The listing builds one solid part. Answer for the finished solid, in the listing's coordinates (mm). A direction names the side the tool comes from. Coordinates: 2 decimals unless noted, no trailing zeros. Loops run counter-clockwise (first coordinate to the right, second up) from the corner with the lowest first, then second, coordinate; pieces in that order, holes last. Notation, with made-up numbers: (-20.75, 32.25) -> (11.25, 32.25) arc R32 cw to (11.25, 68.25) -> close; hole circle Ø2 at (52.25, 55). An arc over 180 degrees is marked (long way). Answer in a Markdown table with one row per item.
```python
from build123d import *

# Parameters (mm, degrees)
F0_W      = 203.2
F0_H      = 203.2
F1_DEPTH  = 203.2
F2_W      = 198.12
F2_H      = 198.12
F3_DEPTH  = 200.66
F7_DEPTH  = 203.201
F10_DEPTH = 2.54
F13_DEPTH = 2.54


with BuildPart() as f1:
    # F0 (on Top) → F1 (new body)
    with BuildSketch(Plane.XY):
        Rectangle(F0_W, F0_H)
    extrude(amount=F1_DEPTH)

    # F2 (on Top) → F3 (cut)
    with BuildSketch(Plane.XY):
        Rectangle(F2_W, F2_H)
    extrude(amount=F3_DEPTH, mode=Mode.SUBTRACT)

    # F6 (on offset) → F7 (cut, through all)
    with BuildSketch(Plane.YZ.offset(101.6)):
        Polygon((1.27, 76.2), (1.27, 101.6), (-99.06, 101.6), (-99.06, 0), (99.06, 0), (99.06, 76.2), align=None)
    extrude(amount=-F7_DEPTH, mode=Mode.SUBTRACT)

    # F9 (on offset) → F10 (cut, through all)
    with BuildSketch(Plane(origin=(0, 101.6, 0), x_dir=(-1, 0, 0), z_dir=(0, 1, 0))):
        Polygon((-101.6, 0), (101.6, 0), (101.6, 25.4), (101.6, 50.8), (50.8, 50.8), (50.8, 25.4), (-50.8, 25.4), (-50.8, 50.8), (-101.6, 50.8), (-101.6, 25.4), align=None)
    extrude(amount=-F10_DEPTH, mode=Mode.SUBTRACT)

    # F12 (on offset) → F13 (cut, through all)
    with BuildSketch(Plane.XZ.offset(101.6)):
        Polygon((-101.6, 101.6), (-101.6, 0), (101.6, 0), (101.6, 101.6), (76.2, 101.6), (76.2, 127), (25.4, 127), (25.4, 101.6), (25.4, 76.2), (-25.4, 76.2), (-25.4, 101.6), (-25.4, 127), (-76.2, 127), (-76.2, 101.6), align=None)
    extrude(amount=-F13_DEPTH, mode=Mode.SUBTRACT)


solid = f1.part
```
Item 1: A cutting plane is placed at B-B, the plane x = 87.5. Determine the outline of the cut face in (y, z), plus the area to 3 significant figures.
Findings below:
| item | result |
|---|---|
| outline | (-101.6, 101.6) -> (-99.06, 101.6) -> (-99.06, 200.66) -> (99.06, 200.66) -> (99.06, 50.8) -> (101.6, 50.8) -> (101.6, 203.2) -> (-101.6, 203.2) -> close |
| area | 1,150 mm2 |
Item 2: A cutting plane is placed at A-A, the plane z = 123. Determine the outline of the cut face in (x, y), plus the area to 3 significant figures.
Findings below:
| item | result |
|---|---|
| outline | (-101.6, -101.6) -> (-76.2, -101.6) -> (-76.2, -99.06) -> (-99.06, -99.06) -> (-99.06, 99.06) -> (99.06, 99.06) -> (99.06, -99.06) -> (76.2, -99.06) -> (76.2, -101.6) -> (101.6, -101.6) -> (101.6, 101.6) -> (-101.6, 101.6) -> close; (-25.4, -101.6) -> (25.4, -101.6) -> (25.4, -99.06) -> (-25.4, -99.06) -> close |
| area | 1,780 mm2 |
Item 3: Find the intervals of material crossed by probe 1 along Y at (x, z) = (14, 177); probe 2 along Z at (x, y) = (82.5, 59), in increasing order.
Findings below:
| item | result |
|---|---|
| probe 1 | y = -101.6 to -99.06, 99.06 to 101.6 |
| probe 2 | z = 200.66 to 203.2 |
Item 4: A cutting plane is placed at D-D, the plane z = 88. Determine the outline of the cut face in (x, y).
Findings below:
| item | result |
|---|---|
| outline | (-101.6, 1.27) -> (-99.06, 1.27) -> (-99.06, 99.06) -> (99.06, 99.06) -> (99.06, 1.27) -> (101.6, 1.27) -> (101.6, 101.6) -> (-101.6, 101.6) -> close; (-25.4, -101.6) -> (25.4, -101.6) -> (25.4, -99.06) -> (-25.4, -99.06) -> close |
Item 5: Determine the mould class of faces 5 (the face through (-101.6, -1, 143)), 6 (the face through (-1, 101.6, 113)), 7 (the face through (99.06, -1, 138)), 8 (the face through (101.6, -1, 143)) for opening direction X: +X half, -X half, draft (parallel to the pull), parting line (faces both ways), or undercut.
Findings below:
| item | result |
|---|---|
| face 5 | -X half |
| face 6 | draft |
| face 7 | undercut |
| face 8 | +X half |
Item 6: Flat-ended cylindrical pins translate along their axes: pin 1 Ø0.8 at (x, y) = (3, -100) entering from -Z; pin 2 Ø12.5 at (x, y) = (-83.5, -55.5) entering from -Z; pin 3 Ø0.8 at (y, z) = (-100.5, 94.5) entering from +X. Find the tip coordinate at first contact, or state that the pin passes through.
Findings below:
| item | result |
|---|---|
| pin 1 | stops at z = 76.2 |
| pin 2 | stops at z = 200.66 |
| pin 3 | stops at x = 25.4 |
Item 7: A cutting plane is placed at C-C, the plane y = 7. Determine the outline of the cut face in (x, z), plus the area to 3 significant figures.
Findings below:
| item | result |
|---|---|
| outline | (-101.6, 76.2) -> (-99.06, 76.2) -> (-99.06, 200.66) -> (99.06, 200.66) -> (99.06, 76.2) -> (101.6, 76.2) -> (101.6, 203.2) -> (-101.6, 203.2) -> close |
| area | 1,150 mm2 |
Item 8: A tool of negligible diameter and unlimited length cuts with its end or side. For faces 1 (the face through (1, 99.06, 112)), 2 (the face through (99.3, -61.8, 101.6)), 3 (the face through (-100, -62, 101.6)), 4 (the face through (-1, -101.6, 153)), from which of +Z, -Z, +X, -X, +Y, -Y can it reach the whole face along a straight path? Write none if from no direction.
Findings below:
| item | result |
|---|---|
| face 1 | -Z |
| face 2 | -Z, +X, -Y |
| face 3 | -Z, -X, -Y |
| face 4 | +Z, -Z, +X, -X, -Y |
